from build123d import *

# Parameters (mm, degrees)
SKETCH018_W          = 50
SKETCH018_H          = 18
PAD011_DEPTH         = 4.5
SKETCH019_R          = 1.3375
POCKET006_DEPTH      = 8
POCKET007_DEPTH      = 9.001
SKETCH021_W          = 6.5
SKETCH021_H          = 18
PAD012_DEPTH         = 26
SKETCH022_R          = 1.75
POCKET008_DEPTH      = 0.001
POCKET008_DEPTH_BACK = 50.001
SKETCH023_R          = 3
POCKET009_DEPTH      = 5
SKETCH024_W          = 10
SKETCH024_H          = 9
SKETCH024_R          = 2.5
PAD013_DEPTH         = 6.5


with BuildPart() as part:
    # Sketch018 → Pad011 (new body, symmetric)
    with BuildSketch(Plane.XY):
        with Locations((25, 9)):
            Rectangle(SKETCH018_W, SKETCH018_H)
    extrude(amount=PAD011_DEPTH, both=True)

    # Sketch019 → Pocket006 (cut)
    with BuildSketch(Plane.XZ):
        with Locations((5, 0)):
            Circle(SKETCH019_R)
        with Locations((25, 0)):
            Circle(SKETCH019_R)
        with Locations((45, 0)):
            Circle(SKETCH019_R)
    extrude(amount=-POCKET006_DEPTH, mode=Mode.SUBTRACT)

    # Sketch020 (on Face4 of Pocket006) → Pocket007 (cut, through all)
    with BuildSketch(Plane(origin=(0, 0, -4.5), x_dir=(1, 0, 0), z_dir=(0, 0, -1))):
        Polygon((0, -8), (43.5, -18), (0, -18), align=None)
    extrude(amount=-POCKET007_DEPTH, mode=Mode.SUBTRACT)

    # Sketch021 (on Face4 of Pocket007) → Pad012 (join)
    with BuildSketch(Plane.XY.offset(-4.5)):
        with Locations((46.75, 9)):
            Rectangle(SKETCH021_W, SKETCH021_H)
    extrude(amount=-PAD012_DEPTH)

    # Sketch022 → Pocket008 (cut, two sides)
    with BuildSketch(Plane.YZ) as pocket008_sk:
        with Locations((4, -25)):
            Circle(SKETCH022_R)
        with Locations((4, -10)):
            Circle(SKETCH022_R)
        with Locations((14, -10)):
            Circle(SKETCH022_R)
        with Locations((14, -25)):
            Circle(SKETCH022_R)
    extrude(amount=-POCKET008_DEPTH, mode=Mode.SUBTRACT)
    extrude(pocket008_sk.sketch, amount=POCKET008_DEPTH_BACK, mode=Mode.SUBTRACT)

    # Sketch023 → Pocket009 (cut, symmetric)
    with BuildSketch(Plane.YZ.offset(32)):
        with Locations((4, -10)):
            Circle(SKETCH023_R)
        with Locations((14, -10)):
            Circle(SKETCH023_R)
        with Locations((14, -25)):
            Circle(SKETCH023_R)
        with Locations((4, -25)):
            Circle(SKETCH023_R)
    extrude(amount=POCKET009_DEPTH, both=True, mode=Mode.SUBTRACT)

    # Sketch024 (on Face7 of Pocket009) → Pad013 (join)
    with BuildSketch(Plane.YZ.offset(50)):
        with Locations((-5, -14.5)):
            Rectangle(SKETCH024_W, SKETCH024_H)
        with Locations((-5, -14.5)):
            Circle(SKETCH024_R, mode=Mode.SUBTRACT)
    extrude(amount=-PAD013_DEPTH)


with BuildPart() as part_1:
    # Body005 placement: moved
    add(part.part.moved(Location((75, 6.5, 0))))


solid = part_1.part
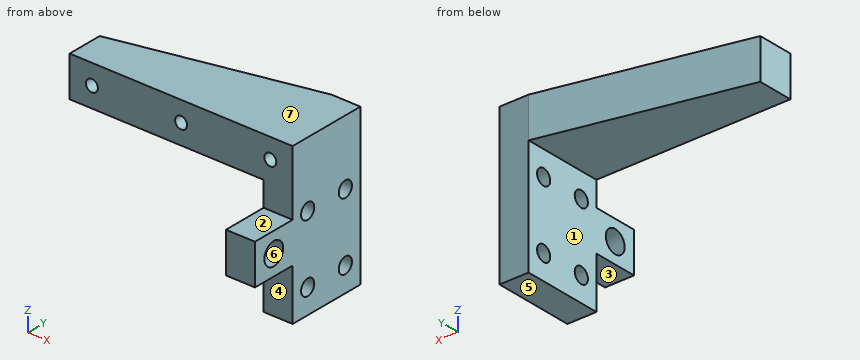
Verification items for the finished model (mm, model axes). Face numbers are marked on the shaded views. A direction names the side the tool comes from. Give positions to 0.01 mm unless a question says otherwise; leave off trailing zeros. Write each loop counter-clockwise with the first axis right and the second up, starting at its lowest first coordinate (ties: lowest second). Pieces come first, ordered by that corner, then holes. Notation, with made-up numbers: M -12,-9.75 L -3,-9.75 A15 cw -3,15.25 Z; hole C -17,44 d3. An arc over 180 degrees is marked long. Put each result on its own line as item: value. Start each with the question number.
1. Section check B-B (z = -14.5). Record the cut outline in (x, y), and give its area (4 significant figures).
2. Section check A-A (y = 10.5). Give the number of separate pieces and of enclosed holes in the cut face, and give its area (3 significant figures).
3. Scan lines: line 1 along Z through (x, y) = (121.75, 10.5); line 2 along Y through (x, z) = (123.5, -25); line 3 along Z through (x, y) = (120, 9.5). Record each from-to range of solid material in increasing order. Write a range as [from, to].
4. Section check D-D (x = 120). Record the cut outline in (y, z), and give its area (3 significant figures).
5. Set-up check for the marked faces 1, 2 and 3: record each of +Z, -Z, +X, -X, +Y, -Y from which the full face is reachable in a straight line by a thin tool's end or side.
6. Go/stop test with flat-tipped pins: pin 1 Ø5.5 at (y, z) = (20.5, -25) entering from -X; pin 2 Ø3.5 at (x, z) = (80, 0) entering from +Y; pin 3 Ø7 at (x, z) = (122.5, -23) entering from -Y. Record where each tip stops, or that it passes through.
7. Draft check along Z on the marked faces 4, 5, 6 and 7. Enter one of: +Z half, -Z half, draft (parallel to the pull), parting line (faces both ways), or undercut.
8. Section check C-C (y = 20.5). Record the cut outline in (x, z).
Answer list:
1. outline: M 118.5,-3.5 L 125,-3.5 L 125,-1 L 118.5,-1 Z; M 118.5,4 L 125,4 L 125,24.5 L 118.5,24.5 Z
1. area: 149.5 mm2
2. separate pieces: 3
2. enclosed holes: 3
2. area: 557 mm2
3. line 1: [-30.5, -26.75], [-23.25, -11.75], [-8.25, 4.5]
3. line 2: [6.5, 8.75], [12.25, 18.75], [22.25, 24.5]
3. line 3: [-30.5, -26.44], [-23.56, -11.44], [-8.56, -1.34], [1.34, 4.5]
4. outline: M -3.5,-19 L 6.5,-19 L 6.5,-30.5 L 24.5,-30.5 L 24.5,4.5 L 6.5,4.5 L 6.5,1.34 L 14.5,1.34 L 14.5,-1.34 L 6.5,-1.34 L 6.5,-10 L -3.5,-10 Z; hole C 1.5,-14.5 d5; hole C 10.5,-25 d3.5; hole C 10.5,-10 d3.5; hole C 20.5,-25 d3.5; hole C 20.5,-10 d3.5
4. area: 640 mm2
5. face 1: -Z, -X, +Y, -Y
5. face 2: +Z, +X, -X, -Y
5. face 3: -Z, +X, -X, -Y
6. pin 1: x = 118.5
6. pin 2: y = 16.05
6. pin 3: y = 6.5
7. face 4: draft
7. face 5: -Z half
7. face 6: undercut
7. face 7: +Z half
8. outline: M 101.1,-4.5 L 118.5,-4.5 L 118.5,-8.25 L 125,-8.25 L 125,4.5 L 101.1,4.5 Z; M 118.5,-30.5 L 125,-30.5 L 125,-26.75 L 118.5,-26.75 Z; M 118.5,-23.25 L 125,-23.25 L 125,-11.75 L 118.5,-11.75 Z
